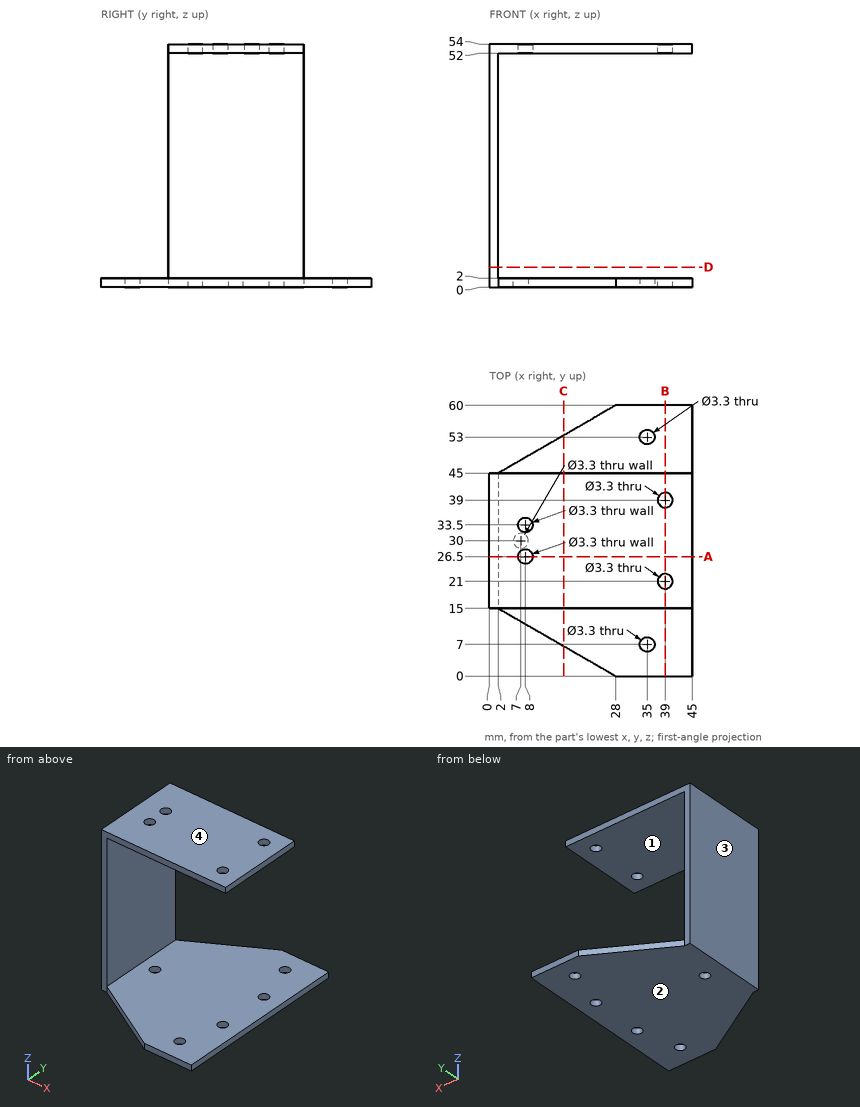
Print and shaded views of the part. All mm, measured from the part's lowest x, y and z. Coordinates: 2 decimals unless noted, no trailing zeros. Order: outer loops, then holes, each group sorted by start corner. A loop starts at its lowest first (then second) coordinate and runs counter-clockwise, first axis right, second up. Notation, with made-up numbers: (-4, 69.25) -> (35, 69.25) arc R29 ccw to (35, 92.25) -> close; hole circle Ø11 at (-33.75, 32.5). An arc over 180 degrees is marked (long way). Use one line per item in the form item = value. Start each with the question number.
1) Band-saw the part on A-A on y = 26.5. Give the cut face in (x, z).
2) Pull direction Z, two halves, no side cores. Call the marked faces 1, 2, 3 and 4: +Z half, -Z half, draft (parallel to the pull), parting line (faces both ways), or undercut.
3) Band-saw the part on B-B on x = 39. Give the cut face in (y, z), then the cut area to 3 significant figures.
4) Drop flat-ended pins along their axis: pin 1 (24 mm diameter, centred on y = 26, z = 29.5, fed in from +X); pin 2 (1 mm diameter, centred on x = 25, y = 46, fed in from +Z). Give the stop position or say it passes through.
5) Band-saw the part on D-D on z = 4.5. Give the cut face in (x, y), then the cut area to 3 significant figures.
6) Band-saw the part on C-C on x = 16.5. Give the cut face in (y, z), then the cut area to 3 significant figures.
7) Drill centre lines: L1, parallel to Y at x = 39, z = 53.5; L2, parallel to Y at x = 8, z = 53.3; L3, parallel to Z at x = 16.5, y = 27. Where is each one in solid material? Low to high. Write a range as [from, to].
Entries:
q1.outline = (0, 0) -> (45, 0) -> (45, 2) -> (2, 2) -> (2, 52) -> (6.35, 52) -> (6.35, 54) -> (0, 54) -> close; (9.65, 52) -> (45, 52) -> (45, 54) -> (9.65, 54) -> close
q2.face_1 = undercut
q2.face_2 = -Z half
q2.face_3 = draft
q2.face_4 = +Z half
q3.outline = (0, 0) -> (19.35, 0) -> (19.35, 2) -> (0, 2) -> close; (15, 52) -> (19.35, 52) -> (19.35, 54) -> (15, 54) -> close; (22.65, 0) -> (37.35, 0) -> (37.35, 2) -> (22.65, 2) -> close; (22.65, 52) -> (37.35, 52) -> (37.35, 54) -> (22.65, 54) -> close; (40.65, 0) -> (60, 0) -> (60, 2) -> (40.65, 2) -> close; (40.65, 52) -> (45, 52) -> (45, 54) -> (40.65, 54) -> close
q3.area = 154 mm2
q4.pin_1 = 2
q4.pin_2 = 2
q5.outline = (0, 15) -> (2, 15) -> (2, 45) -> (0, 45) -> close
q5.area = 60.0 mm2
q6.outline = (6.63, 0) -> (53.37, 0) -> (53.37, 2) -> (6.63, 2) -> close; (15, 52) -> (45, 52) -> (45, 54) -> (15, 54) -> close
q6.area = 153 mm2
q7.L1 = [15, 19.35], [22.65, 37.35], [40.65, 45]
q7.L2 = [15, 24.85], [28.15, 31.85], [35.15, 45]
q7.L3 = [0, 2], [52, 54]
